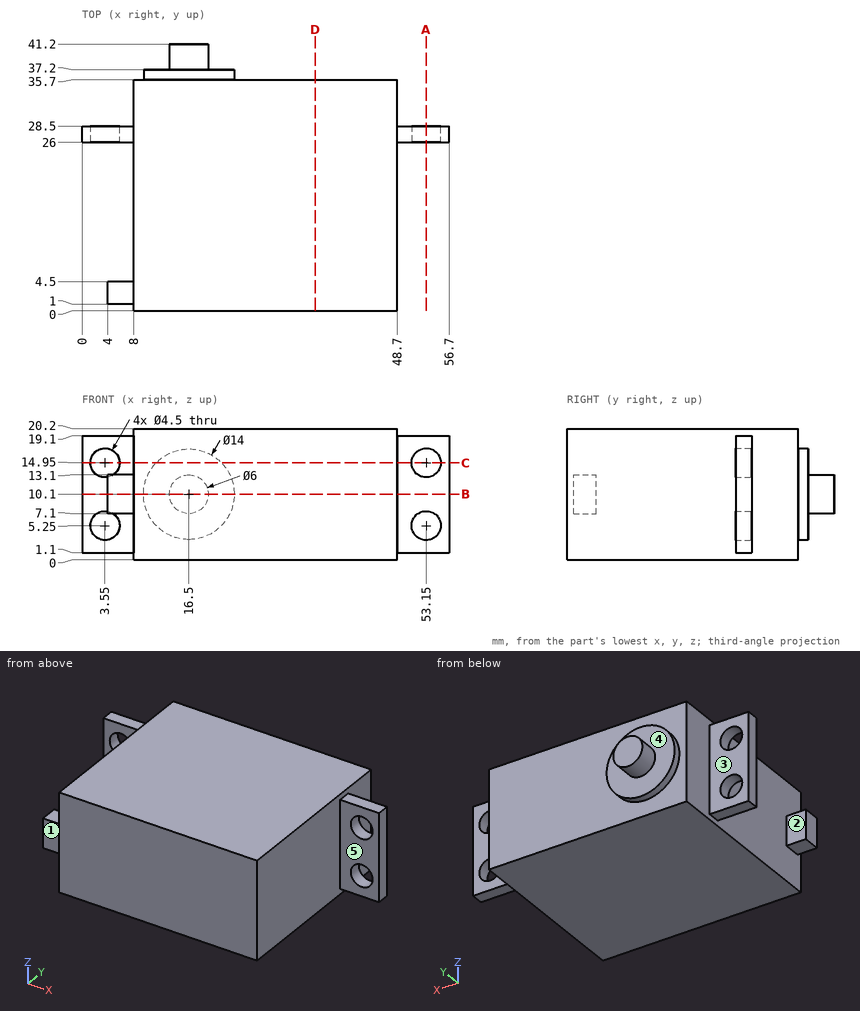
For this review, use the dimensioned drawing (mm, ordinates from the lowest corner) and the shaded views. A direction names the side the tool comes from. Coordinates: 2 decimals unless noted, no trailing zeros. Write each loop counter-clockwise with the first axis right and the second up, starting at its lowest first coordinate (ties: lowest second). Pieces come first, ordered by that corner, then holes. Notation, with made-up numbers: (86.25, -5) - (90.25, -5) arc R23 ccw to (90.25, 8) - close; hole circle Ø7 at (0.5, 75). An arc over 180 degrees is marked (long way). One line per item, written item: value.
1) Add section C-C (z = 14.95). State the section outline as (x, y) points.
Answer sheet:
outline: (0, 26) - (1.3, 26) - (1.3, 28.5) - (0, 28.5) - close; (5.8, 26) - (8, 26) - (8, 0) - (48.7, 0) - (48.7, 26) - (50.9, 26) - (50.9, 28.5) - (48.7, 28.5) - (48.7, 35.7) - (21.55, 35.7) - (21.55, 37.2) - (11.45, 37.2) - (11.45, 35.7) - (8, 35.7) - (8, 28.5) - (5.8, 28.5) - close; (55.4, 26) - (56.7, 26) - (56.7, 28.5) - (55.4, 28.5) - close
2) For the marked faces 1, 2, 3, 4 and 5, list the 3-axis set-ups (+Z, -Z, +X, -X, +Y, -Y) from which the entire face can be reached by the end or side of a thin tool; tool diameter is ignored.
Answer sheet:
face 1: +Z, -Z, -X, -Y
face 2: +Z, -Z, -X
face 3: +Z, -Z, -X, +Y
face 4: +Y
face 5: +Z, -Z, +X, -Y
3) Add section D-D (x = 36). State the section outline as (y, z) points.
Answer sheet:
outline: (0, 0) - (35.7, 0) - (35.7, 20.2) - (0, 20.2) - close
4) Add section A-A (x = 53.15). State the section outline as (y, z) points, plus the area to 3 significant figures.
Answer sheet:
outline: (26, 1.1) - (28.5, 1.1) - (28.5, 3) - (26, 3) - close; (26, 7.5) - (28.5, 7.5) - (28.5, 12.7) - (26, 12.7) - close; (26, 17.2) - (28.5, 17.2) - (28.5, 19.1) - (26, 19.1) - close
area: 22.5 mm2
5) Insertion check: pin 1 (10 mm diameter, centred on x = 10, z = 3, fed in from +Y); pin 2 (3 mm diameter, centred on y = 24, z = 9, fed in from -X); pin 3 (6.5 mm diameter, centred on x = 3.5, z = 14, fed in from -Y); pin 4 (4.5 mm diameter, centred on x = 6.5, z = 10.5, fed in from -Y). Each pin has a flat end and moves straight along its axis. Give the tip position at first contact, or say it passes through.
Answer sheet:
pin 1: stops at y = 37.2
pin 2: stops at x = 8
pin 3: stops at y = 1
pin 4: stops at y = 0
6) To check wall thickness, follow probe 1 along Z at (x, y) = (3.55, 26.8); probe 2 along Z at (x, y) = (3, 27); probe 3 along Y at (x, z) = (7, 7). State the ranges of each line that lie inside material, in increasing order.
Answer sheet:
probe 1: z = 1.1 to 3, 7.5 to 12.7, 17.2 to 19.1
probe 2: z = 1.1 to 3.07, 7.43 to 12.77, 17.13 to 19.1
probe 3: y = 26 to 28.5
7) Add section B-B (z = 10.1). State the section outline as (x, y) points.
Answer sheet:
outline: (0, 26) - (8, 26) - (8, 4.5) - (4, 4.5) - (4, 1) - (8, 1) - (8, 0) - (48.7, 0) - (48.7, 26) - (56.7, 26) - (56.7, 28.5) - (48.7, 28.5) - (48.7, 35.7) - (23.5, 35.7) - (23.5, 37.2) - (19.5, 37.2) - (19.5, 41.2) - (13.5, 41.2) - (13.5, 37.2) - (9.5, 37.2) - (9.5, 35.7) - (8, 35.7) - (8, 28.5) - (0, 28.5) - close
